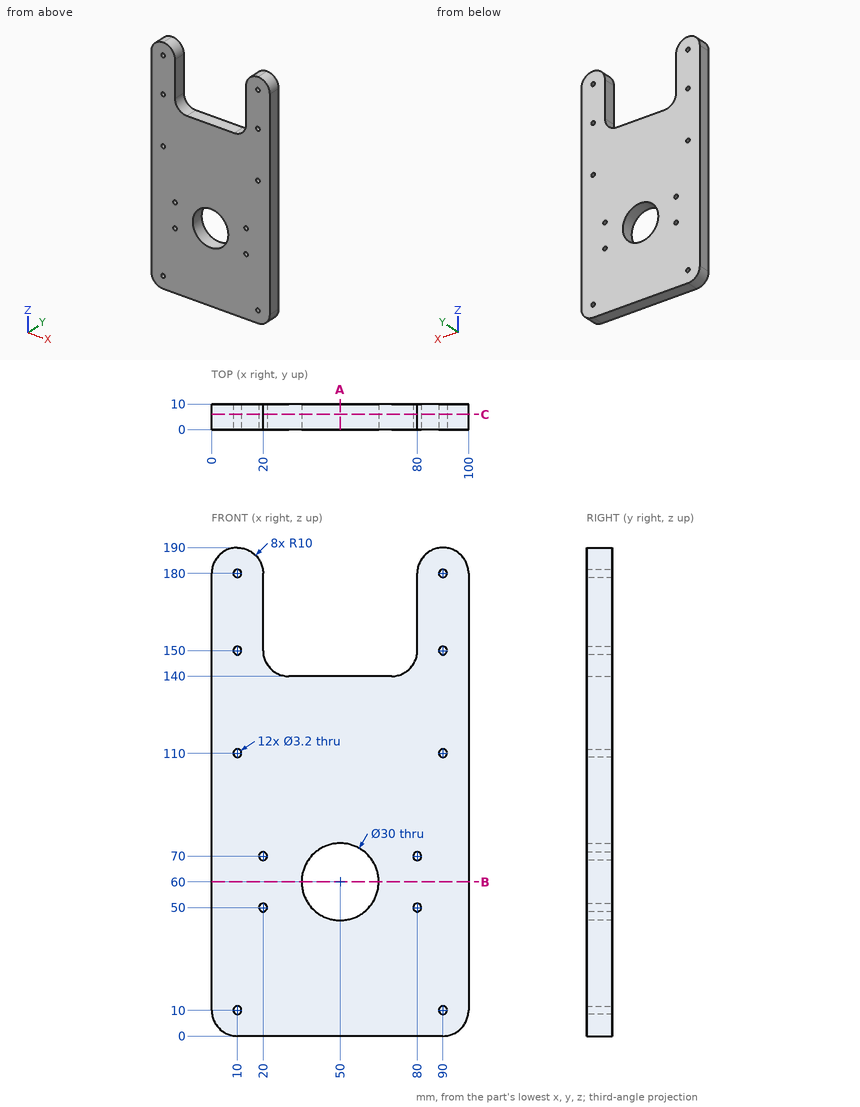
For this review, use the dimensioned drawing (mm, ordinates from the lowest corner) and the shaded views. Coordinates: 2 decimals unless noted, no trailing zeros. Write each loop counter-clockwise with the first axis right and the second up, starting at its lowest first coordinate (ties: lowest second). Pieces come first, ordered by that corner, then holes. Notation, with made-up numbers: (17, -19) - (61, -19) arc R28 cw to (61, 6) - close; hole circle Ø4 at (88.25, 39.5). An arc over 180 degrees is marked (long way). One line per item, written item: value.
1) Add section A-A (x = 50). State the section outline as (y, z) points.
Answer sheet:
outline: (0, 0) - (10, 0) - (10, 45) - (0, 45) - close; (0, 75) - (10, 75) - (10, 140) - (0, 140) - close
2) To check wall thickness, follow probe 1 along X at (y, z) = (7.5, 180); probe 2 along Z at (x, y) = (90, 4.5); probe 3 along Z at (x, y) = (11, 6.75). State the ranges of each line that lie inside material, in increasing order.
Answer sheet:
probe 1: x = 0 to 8.4, 11.6 to 20, 80 to 88.4, 91.6 to 100
probe 2: z = 0 to 8.4, 11.6 to 108.4, 111.6 to 148.4, 151.6 to 178.4, 181.6 to 190
probe 3: z = 0 to 8.75, 11.25 to 108.75, 111.25 to 148.75, 151.25 to 178.75, 181.25 to 189.95
3) Add section C-C (y = 6). Give the number of separate pieces and of enclosed holes in the cut face, plus the area to 3 significant figures.
Answer sheet:
separate pieces: 1
enclosed holes: 13
area: 15,100 mm2
4) Insertion check: pin 1 (2.5 mm diameter, centred on x = 80, z = 50, fed in from +Y); pin 2 (6 mm diameter, centred on x = 25.5, y = 3.5, fed in from +Z); pin 3 (3.5 mm diameter, centred on x = 20, z = 50, fed in from -Y). Each pin has a flat end and moves straight along its axis. Give the tip position at first contact, or say it passes through.
Answer sheet:
pin 1: passes through
pin 2: stops at z = 143.39
pin 3: stops at y = 0
5) Add section B-B (z = 60). State the section outline as (x, y) points, plus the area to 3 significant figures.
Answer sheet:
outline: (0, 0) - (35, 0) - (35, 10) - (0, 10) - close; (65, 0) - (100, 0) - (100, 10) - (65, 10) - close
area: 700 mm2
